Build history of the part. All positions in model axes, mm. Round coordinates to 2 decimals unless told otherwise and drop trailing zeros. Put each result on its own line as item: value. Start each with the question number.
Item 1: Drill centre lines: probe 1 along X at (y, z) = (5.75, -20); probe 2 along X at (y, z) = (5, -346.5); probe 3 along Z at (x, y) = (-169, 5.25). Where is each one in solid material? Low to high. Write a range as [from, to].
Item 2: Pull direction Z, two halves, no side cores. Call faces 1 (the flat face through (-173, 0, -237)), 2 (the cylindrical face through (-3.01, 5.07, -2.85)), 3 (the cylindrical face through (-346.99, 5.07, -477.15)), 4 (the cylindrical face through (-23.794, 7.116, -72.419)): +Z half, -Z half, draft (parallel to the pull), parting line (faces both ways), or undercut.
Item 3: Flat gauge pins, fed straight in: pin 1 Ø3 at (x, z) = (-221.5, -406) entering from -Y; pin 2 Ø10.5 at (x, z) = (-20, -270) entering from -Y; pin 3 Ø11.5 at (x, z) = (-20, -70) entering from -Y. Where does each tip first touch, or does it go through?
Autodesk Inventor part; units mm, degrees
ref_plane "YZ Plane" through (0, 0, 0) normal (1, 0, 0) x (0, 1, 0)
ref_plane "XZ Plane" through (0, 0, 0) normal (0, 1, 0) x (-1, 0, 0)
ref_plane "XY Plane" through (0, 0, 0) normal (0, 0, 1) x (1, 0, 0)
sketch "Sketch1" plane through (0, 0, 0) normal (0, 1, 0) x (-1, 0, 0)
  line L0 (0, 0) -> (350, 0)
  line L1 (350, 0) -> (350, -480)
  line L2 (350, -480) -> (0, -480)
  line L3 (0, -480) -> (0, 0)
  dimension "d0" = 480
  dimension "d1" = 350
extrude "Extrusion1" add sketch "Sketch1" along normal blind 10
fillet "Fillet1" radius 10 4 edges at (-350, 5, 0) (0, 5, 0) (0, 5, -480) (-350, 5, -480)
sketch "Sketch5" plane through (0, 0, 0) normal (0, 1, 0) x (-1, 0, 0)
  line L0 (340, 0) -> (10, 0)
  line L1 (0, -10) -> (0, -470)
  line L2 (20, -70) -> (20, -170) construction
  line L3 (20, -120) -> (20, -220) construction
  line L4 (20, -170) -> (20, -270) construction
  line L5 (20, -20) -> (120, -20) construction
  line L6 (20, -20) -> (20, -120) construction
  line L7 (170, -20) -> (70, -20) construction
  point P0 (0, 0)
  dimension "d32" = 100
  dimension "d33" = 70
  dimension "d34" = 20
  dimension "d43" = 50
hole "Hole4" at (-170, 0, -20) at (-120, 0, -20) at (-70, 0, -20) at (-20, 0, -20) at (-20, 0, -70) at (-20, 0, -120) at (-20, 0, -170) at (-20, 0, -220) at (-20, 0, -270) direction (0, 1, 0) diameter 9 end through all countersink diameter 17.3 countersink angle 90
sketch "Sketch2" plane through (0, 0, 0) normal (0, 1, 0) x (-1, 0, 0)
  line L0 (0, -10) -> (0, -470)
  line L1 (10, -480) -> (340, -480)
  line L2 (88.75, -311.5) -> (108.75, -311.5) construction
  line L3 (108.75, -311.5) -> (128.75, -311.5) construction
  line L4 (108.75, -311.5) -> (112.75, -346.5) construction
  line L5 (45, -346.5) -> (112.75, -346.5) construction
  line L6 (180.5, -346.5) -> (112.75, -346.5) construction
  point P0 (0, 0)
  point P1 (45, -390)
  point P2 (180.5, -390)
  point P3 (128.75, -290.5)
  dimension "d20" = 43.5
  dimension "d21" = 135.5
  dimension "d22" = 45
  dimension "d23" = 90
  dimension "d26" = 40
  dimension "d28" = 21
  dimension "d30" = 35
  dimension "d31" = 4
hole "Hole5" at (-128.75, 0, -290.5) at (-88.75, 0, -311.5) at (-180.5, 0, -346.5) at (-180.5, 0, -390) at (-45, 0, -346.5) at (-45, 0, -390) direction (0, 1, 0) diameter 2.459 end through all
sketch "Sketch3" plane through (0, 0, 0) normal (0, 1, 0) x (-1, 0, 0)
  line L0 (350, -470) -> (350, -10) construction
  line L1 (350, -20) -> (330, -20) construction
  line L2 (330, -20) -> (330, 0) construction
  line L3 (0, -10) -> (0, -470) construction
  line L4 (0, -20) -> (20, -20) construction
  line L5 (20, -20) -> (20, 0) construction
  line L6 (340, 0) -> (10, 0) construction
  line L7 (0, -460) -> (20, -460) construction
  line L8 (20, -460) -> (20, -480) construction
  line L9 (10, -480) -> (340, -480) construction
  line L10 (330, -480) -> (330, -460) construction
  line L11 (330, -460) -> (350, -460) construction
  point P0 (0, 0)
  dimension "d12" = 20
properties part number "bottom_plate" material "Acetal Resin, White"
Reply:
1. probe 1: x = [-350, -174.5], [-165.5, -124.5], [-115.5, -74.5], [-65.5, -24.5], [-15.5, 0]
1. probe 2: x = [-350, -181.73], [-179.27, -46.23], [-43.77, 0]
1. probe 3: z = [-480, -24.39], [-15.61, 0]
2. face 1: draft
2. face 2: +Z half
2. face 3: -Z half
2. face 4: undercut
3. pin 1: stops at y = 0
3. pin 2: stops at y = 3.4
3. pin 3: stops at y = 2.9
